```python
from build123d import *

# Parameters (mm, degrees)
CHAMFER1_SIZE      = 0.6
CUT_EXTRUDE1_DEPTH = 2


with BuildPart() as part:
    # Sketch1 → Revolve1 (revolve)
    with BuildSketch(Plane.XY):
        with BuildLine():
            Line((0, 0), (76.3, 0))
            Line((76.3, 0), (76.3, 3))
            Line((76.3, 3), (2.3, 3))
            Line((2.3, 3), (2.3, 5.7))
            Line((2.3, 5.7), (1.6, 5.7))
            ThreePointArc((1.6, 5.7), (0.632383618, 4.374431764), (0, 2.86))
            Line((0, 2.86), (0, 0))
        make_face()
    revolve(axis=Axis((0, 0, 0), (1, 0, 0)))

    # Chamfer1
    chamfer1_edges = [part.edges().sort_by_distance(p)[0] for p in [
        (76.3, -3, 0),
    ]]
    chamfer(chamfer1_edges, length=CHAMFER1_SIZE)

    # Sketch2 → Cut-Extrude1 (cut)
    with BuildSketch(Plane.ZY):
        Polygon((0, 2.309401077), (-2, 1.154700538), (-2, -1.154700538), (0, -2.309401077), (2, -1.154700538), (2, 1.154700538), align=None)
    extrude(amount=-CUT_EXTRUDE1_DEPTH, mode=Mode.SUBTRACT)


solid = part.part
```
Geometry check sheet. Reference: the model listing, model coordinates, mm. A direction names the side the tool comes from. Coordinates: 2 decimals unless noted, no trailing zeros. Loops run counter-clockwise (first coordinate to the right, second up) from the corner with the lowest first, then second, coordinate; pieces in that order, holes last.
Item 1: Sectioned sample at A-A, the plane x = 52. Record the boundary of the cut face in (y, z), then the cut area to 3 significant figures.
Item 2: Thickness scan on line 1 (X direction, y = 0.75, z = 0); line 2 (Z direction, x = 43, y = -2.25); line 3 (Z direction, x = 68, y = 0). Record the ranges inside material, lowest first.
Item 3: Release check for a two-part mould opening along Y. For faces 4 (the face through (2, 0, 0)), 5 (the face through (0.99, 1.74, -0.99)), 6 (the face through (0, -2, -1)), 7 (the face through (38, -3, 0)) record: released by +Y, released by -Y, zero draft, split by the parting line, or undercut.
Item 4: Access from +Z, -Z, +X, -X, +Y, -Y to the whole of each face (thin tool, end or side, straight path). Record for faces 1 (the face through (2.3, -2.5, -2.5)), 2 (the face through (1.9, -4.5, -3.5)), 3 (the face through (0.986, 1.724, 1.014)).
Item 5: Go/stop test with flat-tipped pins: pin 1 Ø1 at (x, z) = (56.5, -0.5) entering from +Y; pin 2 Ø2 at (x, y) = (0.5, 0) entering from -Z; pin 3 Ø4 at (x, z) = (57.5, -4) entering from +Y. Record where each tip stops, or that it passes through.
Check result:
1. outline: circle Ø6 at (0, 0)
1. area: 28.3 mm2
2. line 1: x = 2 to 76.3
2. line 2: z = -1.98 to 1.98
2. line 3: z = -3 to 3
3. face 4: undercut
3. face 5: undercut
3. face 6: zero draft
3. face 7: split by the parting line
4. face 1: +X
4. face 2: +X, -X
4. face 3: -X
5. pin 1: stops at y = 3
5. pin 2: stops at z = -5.59
5. pin 3: stops at y = 2.24
